```python
from build123d import *

# Parameters (mm, degrees)
F0_W     = 120
F0_H     = 120
F1_DEPTH = 30
F2_R     = 35
F3_DEPTH = 25
F4_R     = 25
F5_DEPTH = 55.001
F6_R     = 1.5
F7_R     = 5
F8_T     = -2


with BuildPart() as f1:
    # F0 (on Front) → F1 (new body)
    with BuildSketch(Plane.XZ):
        with Locations((60, 60)):
            Rectangle(F0_W, F0_H)
    extrude(amount=F1_DEPTH)

    # F2 (on face) → F3 (join)
    with BuildSketch(Plane.XZ.offset(30)):
        with Locations((60, 60)):
            Circle(F2_R)
    extrude(amount=F3_DEPTH)

    # F4 (on face) → F5 (cut, through all)
    with BuildSketch(Plane.XZ.offset(55)):
        with Locations((60, 60)):
            Circle(F4_R)
    extrude(amount=-F5_DEPTH, mode=Mode.SUBTRACT)

    # F6
    f6_edges = [f1.edges().sort_by_distance(p)[0] for p in [
        (35, -55, 60),
        (25, -55, 60),
    ]]
    fillet(f6_edges, radius=F6_R)

    # F7
    f7_edges = [f1.edges().sort_by_distance(p)[0] for p in [
        (25, -30, 60),
        (120, -15, 120),
        (120, -30, 60),
        (60, -30, 120),
        (0, -15, 120),
        (120, -15, 0),
        (60, -30, 0),
        (0, -15, 0),
        (0, -30, 60),
    ]]
    fillet(f7_edges, radius=F7_R)

    # F8
    f8_openings = [f1.faces().sort_by_distance(p)[0] for p in [
        (1.697056, 0, 60),
    ]]
    offset(amount=F8_T, openings=f8_openings)


solid = f1.part
```
Part model, mm, in its own coordinate system. A direction names the side the tool comes from. Coordinates: 2 decimals unless noted, no trailing zeros. Order: outer loops, then holes, each group sorted by start corner. A loop starts at its lowest first (then second) coordinate and runs counter-clockwise, first axis right, second up. Notation, with made-up numbers: (-25, -28) - (-5, -28) arc R22 ccw to (-5, -19) - close; hole circle Ø2 at (35, 78.5). An arc over 180 degrees is marked (long way). Return JSON: item names as keys, results as strings. Group by question number.
Item 1: Which spindle directions (+Z, -Z, +X, -X, +Y, -Y) get a long thin tool onto all of the face, cutting with end or side? Do faces 5 (the face through (1, -28, 61)), 6 (the face through (35, -28, 97)), 7 (the face through (55.44, -44.12, 94.7)). Say none if no direction does.
Item 2: Cut at C-C (y = -40). List the corners of the cut face in (x, z), plus the area to 3 significant figures.
Item 3: Pull direction X, two halves, no side cores. Call faces 1 (the face through (118, -13, 119)), 2 (the face through (35, -30, 97)), 3 (the face through (47.6, -53, 35.7)), 4 (the face through (60.77, -27.1, 2.86)): pulls with the +X half, pulls with the -X half, needs draft (parallel to the pull), parting line crosses it, or undercut.
Item 4: Drill centre lines: probe 1 along Z at (x, y) = (60, -39); probe 2 along X at (y, z) = (-5.5, 78); probe 3 along Z at (x, y) = (60, -29). Where is each one in solid material? Low to high. Write a range as from..to.
Item 5: Cut at B-B (z = 106). List the corners of the cut face in (x, y), plus the area to 3 significant figures.
Item 6: Pin check, flat tips, straight feed: pin 1 (8 mm diameter, centred on x = 25, z = 21.5, fed in from +Y); pin 2 (3 mm diameter, centred on y = -29.5, z = 72.5, fed in from +X); pin 3 (5 mm diameter, centred on x = 86.5, y = -39, fed in from +Z). Stop position of each tip, or through.
Item 7: Cut at A-A (y = -7.5). List the corners of the cut face in (x, z).
Check values:
{
 "1": {"face 5": "+Z, -Z, -X, -Y", "face 6": "+Y", "face 7": "-Y"},
 "2": {"outline": "circle Ø70 at (60, 60); circle Ø54 at (60, 60); hole circle Ø66 at (60, 60); hole circle Ø50 at (60, 60)", "area": "754 mm2"},
 "3": {"face 1": "pulls with the +X half", "face 2": "needs draft", "face 3": "undercut", "face 4": "undercut"},
 "4": {"probe 1": "z = 25..27, 33..35, 85..87, 93..95", "probe 2": "x = 0..2, 39.88..42.65, 77.35..80.12, 118..120", "probe 3": "z = 2..23.61, 33..35, 85..87, 96.39..118"},
 "5": {"outline": "(0, -25) arc R5 ccw to (5, -30) - (115, -30) arc R5 ccw to (120, -25) - (120, 0) - (118, 0) - (118, -25) arc R3 cw to (115, -28) - (5, -28) arc R3 cw to (2, -25) - (2, 0) - (0, 0) - close", "area": "345 mm2"},
 "6": {"pin 1": "stops at y = -28", "pin 2": "stops at x = 119", "pin 3": "stops at z = 85.48"},
 "7": {"outline": "(0, 5) arc R5 ccw to (5, 0) - (115, 0) arc R5 ccw to (120, 5) - (120, 115) arc R5 ccw to (115, 120) - (5, 120) arc R5 ccw to (0, 115) - close; circle Ø54 at (60, 60); hole (2, 5) arc R3 ccw to (5, 2) - (115, 2) arc R3 ccw to (118, 5) - (118, 115) arc R3 ccw to (115, 118) - (5, 118) arc R3 ccw to (2, 115) - close; hole circle Ø50 at (60, 60)"}
}
